Geometry check sheet. Reference: the model listing, model coordinates, mm. Round coordinates to 2 decimals unless told otherwise and drop trailing zeros. Write each loop counter-clockwise with the first axis right and the second up, starting at its lowest first coordinate (ties: lowest second). Pieces come first, ordered by that corner, then holes.
Item 1: Cross-section at A-A (z = 0). Enter the section's corners in (x, y) (3 decimals).
Item 2: Scan lines: probe 1 along Z at (x, y) = (4.5, 1.75); probe 2 along Z at (x, y) = (5, 1.5). Record each from-to range of solid material in increasing order.
Item 3: Depth check by flat-ended pin: P1, Ø4, axis at x = 2.5, y = 6, coming from the +Z side; P2, Ø1, axis at x = -4, y = 4, coming from the +Z side. Enter the tip coordinate at first touch or a pass-through.
Item 4: Cross-section at B-B (x = 0). Enter the section's corners in (y, z) (3 decimals), then the cut area to 3 significant figures.
Autodesk Fusion 360 part; units mm, degrees
sketch "Sketch1" plane through (0, 0, 0) normal (0, 1, 0) x (1, 0, 0)
  circle A0 centre (0, 0) radius 5.715
  dimension "d3" = 11.43
extrude "Extrude1" add sketch "Sketch1" along normal blind 8.001 makes body 1
chamfer "Chamfer1" distance 1.27 angle 45 1 edges at (-5.3283, 8.001, 2.0666) on bodies 1
copy_body "Body->Comp1" bodies 1 removing the originals makes body 2 in component "Peg"
component "Peg" placed x (1, 0, 0) y (0, 1, 0) z (0, 0, 1) at (0, 0, 0)
equation "pegDiameter = 0.45 in"
equation "pegDepth = 0.2 in + boardThickness"
equation "d3 = pegDiameter"
equation "d4 = pegDepth"
equation "boardThickness = 0.115 in"
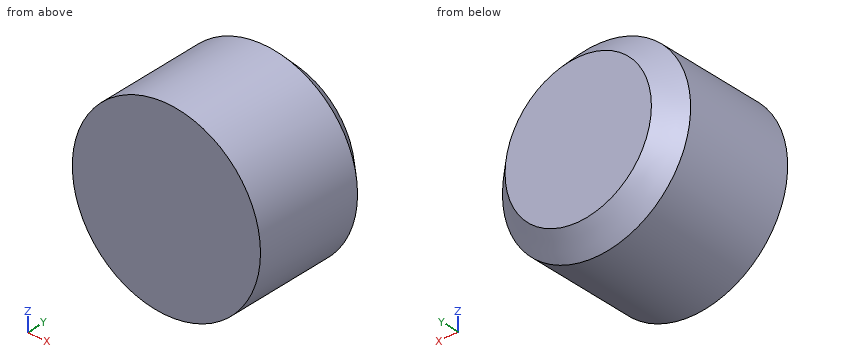
Resolved:
1. outline: (-5.715, 0) - (5.715, 0) - (5.715, 6.731) - (4.445, 8.001) - (-4.445, 8.001) - (-5.715, 6.731) - close
2. probe 1: z = -3.52 to 3.52
2. probe 2: z = -2.77 to 2.77
3. P1: stops at z = 5.69
3. P2: stops at z = 4.52
4. outline: (0, -5.715) - (6.731, -5.715) - (8.001, -4.445) - (8.001, 4.445) - (6.731, 5.715) - (0, 5.715) - close
4. area: 89.8 mm2
